Read the model definition and answer for the solid it produces. Units are mm, in the model's axes. A direction names the side the tool comes from. Coordinates: 2 decimals unless noted, no trailing zeros. Write each loop counter-clockwise with the first axis right and the second up, starting at its lowest first coordinate (ties: lowest second). Pieces come first, ordered by that corner, then holes.
(1) Section A-A on z = 0.55 is taken. Write down the section's boundary in (x, y), then the cut area to 3 significant figures.
(2) Which of the six approach directions +Z, -Z, +X, -X, +Y, -Y give full straight-line access (tool end or side, diameter ignored) to faces 1 (the flat face through (-8, -23.2, 2.5)), 2 (the flat face through (0, -22.75, 1)), 3 (the cylindrical face through (-8.09, -15.15, 1.01)), 4 (the flat face through (8, -23.3, 2.5))?
(3) Section B-B on y = 2.5 is taken. Write down the section's boundary in (x, z), then the cut area to 3 significant figures.
(4) Section C-C on x = -5 is taken. Write down the section's boundary in (y, z).
(5) Find the intervals of material crossed by probe 1 along Z at (x, y) = (-14, 9.5); probe 2 along Y at (x, z) = (-0.5, 0.45); probe 3 along X at (y, z) = (7.5, 2.85), in increasing order.
(6) Given pin 1 (0.5 mm diameter, centred on y = -23.5, z = 2.5, fed in from +X); pin 2 (1.5 mm diameter, centred on x = 8, z = 2, fed in from +Y); pin 3 (1.6 mm diameter, centred on x = -3.5, z = 0.5, fed in from -Y), each flat-ended and moving along its own axis, determine where each tip first touches the part or whether it passes through.
from build123d import *

# Parameters (mm, degrees)
F1_DEPTH = 2
F2_R     = 15
F3_R     = 15
F4_W     = 14
F4_H     = 1
F5_DEPTH = 1
F6_R     = 5


with BuildPart() as f1:
    # F0 (on Top) → F1 (new body)
    with BuildSketch(Plane.XY):
        with BuildLine():
            Line((7, -16.75), (7, -13.5485239048))
            ThreePointArc((7, -13.5485239048), (14.8185270784, 3.6019099414), (0, 15.25))
            Line((0, 15.25), (0, -22.75))
            Line((0, -22.75), (7, -22.75))
            Line((7, -22.75), (7, -16.75))
        make_face()
        with BuildLine():
            Line((0, -22.75), (0, 15.25))
            ThreePointArc((0, 15.25), (-14.8185270784, 3.6019099414), (-7, -13.5485239048))
            Line((-7, -13.5485239048), (-7, -16.75))
            Line((-7, -16.75), (-7, -22.75))
            Line((-7, -22.75), (0, -22.75))
        make_face()
    extrude(amount=F1_DEPTH)

    # F2
    f2_edges = [f1.edges().sort_by_distance(p)[0] for p in [
        (-7, -13.548524, 1),
    ]]
    fillet(f2_edges, radius=F2_R)

    # F3
    f3_edges = [f1.edges().sort_by_distance(p)[0] for p in [
        (7, -13.548524, 1),
    ]]
    fillet(f3_edges, radius=F3_R)

    # F4 (on face) → F5 (join)
    with BuildSketch(Plane.XY.offset(2)):
        with BuildLine():
            ThreePointArc((9.62403785, -15.2229276029), (15.7747967541, -8.6899606851), (18.0099869334, 0))
            ThreePointArc((18.0099869334, 0), (-8.6899606851, 15.7747967541), (-9.62403785, -15.2229276029))
            ThreePointArc((-9.62403785, -15.2229276029), (0, -18.0099869334), (9.62403785, -15.2229276029))
        make_face()
        with BuildLine():
            ThreePointArc((9.62403785, -15.2229276029), (0, -18.0099869334), (-9.62403785, -15.2229276029))
            Line((-9.62403785, -15.2229276029), (-7, -22.75))
            Line((-7, -22.75), (7, -22.75))
            Line((7, -22.75), (9.62403785, -15.2229276029))
        make_face()
        Polygon((-7, -22.75), (-9.62403785, -15.2229276029), (-7, -23.75), align=None)
        Polygon((-7, -23.75), (-9.62403785, -15.2229276029), (-8, -22.75), (-8, -23.75), align=None)
        Polygon((7, -23.75), (9.62403785, -15.2229276029), (7, -22.75), align=None)
        Polygon((8, -22.75), (9.62403785, -15.2229276029), (7, -23.75), (8, -23.75), align=None)
        with Locations((0, -23.25)):
            Rectangle(F4_W, F4_H)
    extrude(amount=F5_DEPTH)

    # F6
    f6_edges = [f1.edges().sort_by_distance(p)[0] for p in [
        (9.624038, -15.222928, 2.5),
        (-9.624038, -15.222928, 2.5),
    ]]
    fillet(f6_edges, radius=F6_R)


solid = f1.part
Response:
1. outline: (-11.09, -10.47) arc R15 cw to (-7, -20.76) - (-7, -22.75) - (7, -22.75) - (7, -20.76) arc R15 cw to (11.09, -10.47) arc R15.25 ccw (long way) to start
1. area: 856 mm2
2. face 1: +Z, -Z, -X, -Y
2. face 2: -Z, +X, -X, -Y
2. face 3: -Z, -X, -Y
2. face 4: +Z, -Z, +X, -Y
3. outline: (-17.84, 2) - (-15.04, 2) - (-15.04, 0) - (15.04, 0) - (15.04, 2) - (17.84, 2) - (17.84, 3) - (-17.84, 3) - close
3. area: 95.8 mm2
4. outline: (-23.75, 2) - (-22.75, 2) - (-22.75, 0) - (14.41, 0) - (14.41, 2) - (17.3, 2) - (17.3, 3) - (-23.75, 3) - close
5. probe 1: z = 2 to 3
5. probe 2: y = -22.75 to 15.24
5. probe 3: x = -16.37 to 16.37
6. pin 1: stops at x = 8
6. pin 2: stops at y = 16.49
6. pin 3: stops at y = -22.75
